Design review of the part built by this model. Coordinates are the model's own, in mm. Round coordinates to 2 decimals unless told otherwise and drop trailing zeros. Write each loop counter-clockwise with the first axis right and the second up, starting at its lowest first coordinate (ties: lowest second). Pieces come first, ordered by that corner, then holes. Notation, with made-up numbers: M 58.25,30 L 106.25,30 A20 cw 106.25,53 Z; hole C -14.5,56.25 d10. An arc over 180 degrees is marked long. One line per question, with ' | ' between items. Start each with the question number.
Item 1: For L1, parallel to Z at x = 0, y = 3.5 (3 decimals); L2, parallel to X at y = 9.25, z = 0 (3 decimals), list the stretches that pass through material, from the lowest coordinate up.
Item 2: Draft analysis for pull direction X (two halves, no side actions). For faces 1 (the face through (5.069, 12.946, -1.596)), 2 (the face through (0, 12, 0)), 3 (the face through (1.3, 0, 1.3)), state which applies: released by +X, released by -X, zero draft, split by the parting line, or undercut.
Item 3: Insertion check: pin 1 Ø1.9 at (x, z) = (0, 0) entering from -Y; pin 2 Ø2 at (y, z) = (14, -5.5) entering from +X; pin 3 Ø10 at (x, y) = (2.5, 13) entering from -Z. Each pin has a flat end and moves straight along its axis. Give the tip position at first contact, or say it passes through.
Item 4: Add section A-A, the plane y = 7.5. State the section outline as (x, z) points (3 decimals), and give its area (3 significant figures).
Item 5: Add section B-B, the plane y = 10.75. State the section outline as (x, z) points (3 decimals), and give its area (3 significant figures).
```python
from build123d import *

# Parameters (mm, degrees)
SKETCH1_R           = 3
SKETCH1_R_2         = 1.585
BOSS_EXTRUDE1_DEPTH = 5
FILLET1_R           = 40
SKETCH8_R           = 1.585
CUT_EXTRUDE1_DEPTH  = 7


with BuildPart() as part:
    # Sketch1 → Boss-Extrude1 (new body)
    with BuildSketch(Plane(origin=(0, 0, 0), x_dir=(1, 0, 0), z_dir=(0, 1, 0))):
        Circle(SKETCH1_R)
        Circle(SKETCH1_R_2, mode=Mode.SUBTRACT)
    extrude(amount=BOSS_EXTRUDE1_DEPTH)

    # Sketch4 → Revolve6 (revolve)
    with BuildSketch(Plane.XY):
        Polygon((8.5, 5), (2.085, 21), (0, 21), (0, 5), align=None)
    revolve(axis=Axis((0, 5, 0), (0, 1, 0)))

    # Sketch7 → Revolve7 (revolve)
    with BuildSketch(Plane.XY):
        Polygon((0, 21), (2.085, 21), (0, 24.39818393), align=None)
    revolve(axis=Axis((0, 21, 0), (0, 1, 0)))

    # Fillet1
    fillet1_edges = [part.edges().sort_by_distance(p)[0] for p in [
        (-2.085, 21, 0),
    ]]
    fillet(fillet1_edges, radius=FILLET1_R)

    # Sketch8 → Cut-Extrude1 (cut)
    with BuildSketch(Plane.XZ.offset(-5)):
        Circle(SKETCH8_R)
    extrude(amount=-CUT_EXTRUDE1_DEPTH, mode=Mode.SUBTRACT)


solid = part.part
```
Computed values:
1) L1: z = -3 to -1.585, 1.585 to 3 | L2: x = -6.796 to -1.585, 1.585 to 6.796
2) face 1: split by the parting line | face 2: undercut | face 3: zero draft
3) pin 1: stops at y = 12 | pin 2: stops at x = 2.12 | pin 3: stops at z = -7.14
4) outline: C 0,0 d14.995; hole C 0,0 d3.17 | area: 169 mm^2
5) outline: C 0,0 d12.389; hole C 0,0 d3.17 | area: 113 mm^2
